Source: three-view drawing plus pictorial views. Frame: mm from the lowest corner of the part. A direction names the side the tool comes from. Give positions to 0.01 mm unless a question says otherwise; leave off trailing zeros. Order: outer loops, then holes, each group sorted by start corner. A loop starts at its lowest first (then second) coordinate and runs counter-clockwise, first axis right, second up. Notation, with made-up numbers: M 23,67.5 L 30,67.5 A28 cw 30,103.5 Z; hole C 73,70.25 d1. An arc over 180 degrees is marked long. Use CSV: the item, a comma, the result in double quotes. Start each with the question number.
Item 1: Section query B-B on x = 2. Return loops of the section in (y, z), and give its area (3 significant figures).
Item 2: Section query D-D on z = 5.2. Return loops of the section in (x, y), and give its area (3 significant figures).
Item 3: Access query for the marked faces 1, 2 and 3. Directions: +Z, -Z, +X, -X, +Y, -Y. A direction counts if a zero-diameter tool reaches every point of the face in a straight line with its end or side. Return the directions, or none.
Item 4: Section query A-A on z = 3.85. Return loops of the section in (x, y).
Item 5: First-contact query: pin 1 (1 mm diameter, centred on x = 7, y = 1.5, fed in from -Z); pin 2 (0.6 mm diameter, centred on x = 8.5, y = 3.5, fed in from -Z). Flat tips, straight axial feed; report the tip coordinate or a pass-through.
Item 6: Ray query, probe 1 along X at (y, z) = (0.8, 2.55); probe 2 along X at (y, z) = (3.5, 3); probe 3 along Y at (x, z) = (2, 3.6). Return the intervals inside material, ascending. Write a range as from..to.
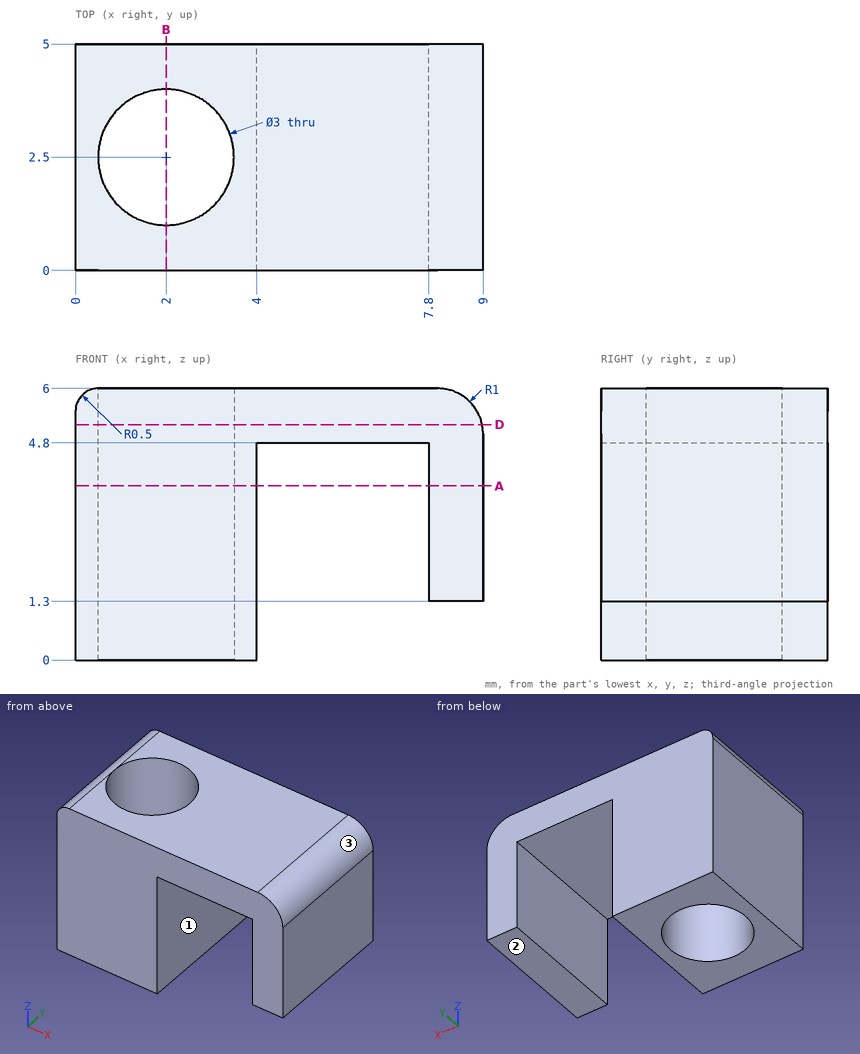
Verdict:
1,outline,"M 0,0 L 1,0 L 1,6 L 0,6 Z; M 4,0 L 5,0 L 5,6 L 4,6 Z"
1,area,"12.0 mm2"
2,outline,"M 0,0 L 8.98,0 L 8.98,5 L 0,5 Z; hole C 2,2.5 d3"
2,area,"37.8 mm2"
3,face 1,"-Z, +Y, -Y"
3,face 2,"-Z, +X, +Y, -Y"
3,face 3,"+Z, +X, +Y, -Y"
4,outline,"M 0,0 L 4,0 L 4,5 L 0,5 Z; M 7.8,0 L 9,0 L 9,5 L 7.8,5 Z; hole C 2,2.5 d3"
5,pin 1,"z = 4.8"
5,pin 2,"z = 1.3"
6,probe 1,"0..4, 7.8..9"
6,probe 2,"0..0.88, 3.12..4, 7.8..9"
6,probe 3,"0..1, 4..5"
